from build123d import *

# Parameters (mm, degrees)
F0_R     = 0.4191
F0_R_2   = 3.175
F1_DEPTH = 3.556
F0_W     = 16.2684546465
F0_H     = 2.54
F0_H_2   = 1.778
F2_DEPTH = 5.969
F3_DEPTH = 1.524
F4_DEPTH = 30.48


with BuildPart() as f1:
    # F0 (on Top) → F1 (new body)
    with BuildSketch(Plane.XY):
        Polygon((-8.1289618026, 19.5699129487), (-8.1289618026, -28.7827895308), (8.1284994147, -28.7827895308), (8.1284994147, 19.5406646823), align=None)
        with Locations((-3.8069129527, -26.3434465483)):
            Circle(F0_R, mode=Mode.SUBTRACT)
        with Locations((3.8130870473, -26.3434465483)):
            Circle(F0_R, mode=Mode.SUBTRACT)
        with BuildLine():
            ThreePointArc((4.0638460346, -14.7540253319), (0.0030865228, -18.8226827446), (-4.0641509764, -14.7605010551))
            Line((-4.0641509764, -14.7605010551), (-4.069773258, -2.185850306))
            ThreePointArc((-4.069773258, -2.185850306), (-3.8099907741, -1.5581196008), (-3.1823557791, -1.2981059663))
            Line((-3.1823557791, -1.2981059663), (-3.1823557791, 8.6078940337))
            Line((-3.1823557791, 8.6078940337), (3.1676447176, 8.6078940337))
            Line((3.1676447176, 8.6078940337), (3.1676447176, -1.2981059659))
            ThreePointArc((3.1676447176, -1.2981059659), (3.7912426345, -1.5606685465), (4.0494391018, -2.1860868505))
            Line((4.0494391018, -2.1860868505), (4.0638460346, -14.7540253319))
        make_face(mode=Mode.SUBTRACT)
        with BuildLine():
            Line((-8.1289618026, -28.7827895308), (-8.1275002277, -38.637912922))
            ThreePointArc((-8.1275002501, -38.637912922), (0.0011022648, -46.764707356), (8.1284994371, -38.6367074901))
            Line((8.1284994147, -38.6367074901), (8.1284994147, -28.7827895308))
            Line((8.1284994147, -28.7827895308), (-8.1289618026, -28.7827895308))
        make_face()
        with Locations((0.0004995041, -37.0354612684)):
            Circle(F0_R_2, mode=Mode.SUBTRACT)
    extrude(amount=F1_DEPTH)

    # F0 (on Top) → F2 (join)
    with BuildSketch(Plane.XY):
        Polygon((-8.1289618026, 25.6512917549), (-8.1289618026, 19.5699129487), (8.1284994147, 19.5406646823), (8.1394928439, 25.6512917549), align=None)
        with Locations((0.0052655206, 26.9212917549)):
            Rectangle(F0_W, F0_H)
        with Locations((0.0052655206, 29.0802917549)):
            Rectangle(F0_W, F0_H_2)
    extrude(amount=F2_DEPTH)

    # F0 (on Top) → F3 (join)
    with BuildSketch(Plane.XY):
        with Locations((0.0052655206, 29.0802917549)):
            Rectangle(F0_W, F0_H_2)
    extrude(amount=-F3_DEPTH)

    # F0 (on Top) → F4 (join)
    with BuildSketch(Plane.XY):
        Polygon((-8.1289618026, 19.5699129487), (-8.1289618026, -28.7827895308), (8.1284994147, -28.7827895308), (8.1284994147, 19.5406646823), align=None)
        with Locations((-3.8069129527, -26.3434465483)):
            Circle(F0_R, mode=Mode.SUBTRACT)
        with Locations((3.8130870473, -26.3434465483)):
            Circle(F0_R, mode=Mode.SUBTRACT)
        with BuildLine():
            ThreePointArc((4.0638460346, -14.7540253319), (0.0030865228, -18.8226827446), (-4.0641509764, -14.7605010551))
            Line((-4.0641509764, -14.7605010551), (-4.069773258, -2.185850306))
            ThreePointArc((-4.069773258, -2.185850306), (-3.8099907741, -1.5581196008), (-3.1823557791, -1.2981059663))
            Line((-3.1823557791, -1.2981059663), (-3.1823557791, 8.6078940337))
            Line((-3.1823557791, 8.6078940337), (3.1676447176, 8.6078940337))
            Line((3.1676447176, 8.6078940337), (3.1676447176, -1.2981059659))
            ThreePointArc((3.1676447176, -1.2981059659), (3.7912426345, -1.5606685465), (4.0494391018, -2.1860868505))
            Line((4.0494391018, -2.1860868505), (4.0638460346, -14.7540253319))
        make_face(mode=Mode.SUBTRACT)
        with BuildLine():
            Line((-4.069773258, -2.185850306), (-4.0641509764, -14.7605010551))
            ThreePointArc((-4.0641509764, -14.7605010551), (0.0030865228, -18.8226827446), (4.0638460346, -14.7540253319))
            Line((4.0638460346, -14.7540253319), (4.0494391018, -2.1860868505))
            ThreePointArc((4.0494391018, -2.1860868505), (3.7912426345, -1.5606685465), (3.1676447176, -1.2981059659))
            Line((3.1676447176, -1.2981059659), (3.1676447176, 8.6078940337))
            Line((3.1676447176, 8.6078940337), (-3.1823557791, 8.6078940337))
            Line((-3.1823557791, 8.6078940337), (-3.1823557791, -1.2981059663))
            ThreePointArc((-3.1823557791, -1.2981059663), (-3.8099907741, -1.5581196008), (-4.069773258, -2.185850306))
        make_face()
        Polygon((-8.1289618026, 25.6512917549), (-8.1289618026, 19.5699129487), (8.1284994147, 19.5406646823), (8.1394928439, 25.6512917549), align=None)
        with Locations((3.8130870473, -26.3434465483)):
            Circle(F0_R)
        with Locations((-3.8069129527, -26.3434465483)):
            Circle(F0_R)
    extrude(amount=-F4_DEPTH)


solid = f1.part
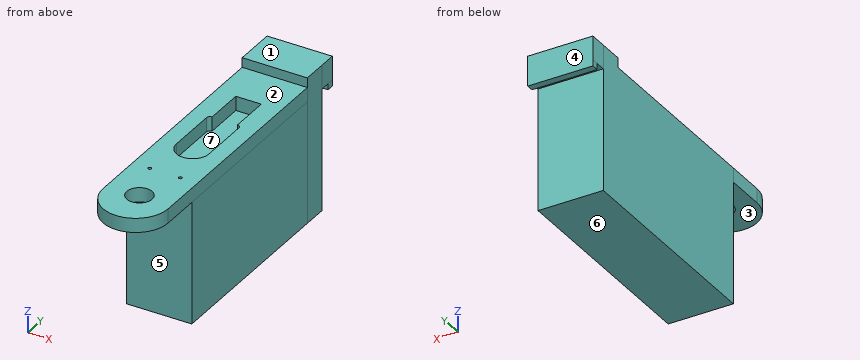
Input: part model. Units: mm. Frame: model coordinates. Face numbers are marked on the shaded views. A direction names the side the tool comes from. Give positions to 0.01 mm unless a question says otherwise; leave off trailing zeros. Order: outer loops, then holes, each group sorted by start corner. A loop starts at its lowest first (then second) coordinate and runs counter-clockwise, first axis right, second up.
Q1. Contact query for flat-ended pins moving along their axis: pin 1 Ø6 at (x, z) = (3, -1.5) entering from -Y; pin 2 Ø8 at (x, z) = (0, -16.5) entering from -Y; pin 3 Ø1 at (y, z) = (-16, 1.5) entering from +X; pin 4 Ø5.5 at (x, y) = (0, -37.04) entering from -Z. Output: stop coordinate, or through.
Checked values:
pin 1: stops at y = -46.75
pin 2: stops at y = -28.78
pin 3: stops at x = 8.13
pin 4: passes through
Q2. Set-up query: the marked faces 1, 2 and 3. Return all of +Z, -Z, +X, -X, +Y, -Y with unobstructed straight access to the full face (end or side cutting, diameter ignored); none if empty.
Checked values:
face 1: +Z, +X, -X, +Y, -Y
face 2: +Z, +X, -X, -Y
face 3: -Z, +X, -X, -Y
Q3. Section B-B on x = -2. Output: boundary loops of the cut face in (y, z), and give its area (3 significant figures).
Checked values:
outline: (-46.51, 0) - (-39.5, 0) - (-39.5, 3.56) - (-46.51, 3.56) - close; (-34.57, 0) - (-28.78, 0) - (-28.78, -30.48) - (25.65, -30.48) - (25.65, 0) - (28.19, 0) - (28.19, -1.52) - (29.97, -1.52) - (29.97, 5.97) - (19.56, 5.97) - (19.56, 3.56) - (8.61, 3.56) - (8.61, 0) - (-18.3, 0) - (-18.3, 3.56) - (-34.57, 3.56) - close
area: 1,850 mm2
Q4. Section A-A on z = 1.5. State how many separate pieces and enclosed holes the cut face has, and give its area (3 significant figures).
Checked values:
separate pieces: 1
enclosed holes: 4
area: 989 mm2
Q5. Section D-D on x = 7.25. Output: boundary loops of the cut face in (y, z).
Checked values:
outline: (-42.31, 0) - (-28.78, 0) - (-28.78, -30.48) - (25.65, -30.48) - (25.65, 0) - (28.19, 0) - (28.19, -1.52) - (29.97, -1.52) - (29.97, 5.97) - (19.54, 5.97) - (19.54, 3.56) - (-42.31, 3.56) - close
Q6. Section C-C on y = -6. Output: boundary loops of the cut face in (x, z).
Checked values:
outline: (-8.13, -30.48) - (8.13, -30.48) - (8.13, 3.56) - (4.05, 3.56) - (4.05, 0) - (-4.07, 0) - (-4.07, 3.56) - (-8.13, 3.56) - close
Q7. Draft query along Y for the marked faces 4, 5, 6 and 7. Return one class per face: +Y half, -Y half, draft (parallel to the pull), parting line (faces both ways), or undercut.
Checked values:
face 4: +Y half
face 5: -Y half
face 6: draft
face 7: undercut
Q8. Ray query, probe 1 along X at (y, z) = (-12.5, 2.5); probe 2 along Y at (x, z) = (1, 2); probe 3 along X at (y, z) = (-26, -6). Return the intervals inside material, ascending.
Checked values:
probe 1: x = -8.13 to -4.07, 4.06 to 8.13
probe 2: y = -46.7 to -40.05, -34.02 to -18.7, 8.61 to 29.97
probe 3: x = -8.13 to 8.13
